from build123d import *

# Parameters (mm, degrees)
SKETCH1_R               = 10
BOSS_EXTRUDE1_DEPTH     = 25
CUT_EXTRUDE2_DEPTH      = 257.353271873
CUT_EXTRUDE2_DEPTH_BACK = 257.353271873
SKETCH3_W               = 67
SKETCH3_H               = 15


with BuildPart() as part:
    # Sketch1 → Boss-Extrude1 (new body)
    with BuildSketch(Plane.XY):
        with BuildLine():
            Line((-230, 24), (230, 24))
            ThreePointArc((230, 24), (254, 0), (230, -24))
            Line((230, -24), (-230, -24))
            ThreePointArc((-230, -24), (-254, 0), (-230, 24))
        make_face()
        with Locations((-230, 0)):
            Circle(SKETCH1_R, mode=Mode.SUBTRACT)
        with Locations(Location((230, 0, 0), (0, 0, 180))):
            Circle(SKETCH1_R, mode=Mode.SUBTRACT)
    extrude(amount=-BOSS_EXTRUDE1_DEPTH)

    # Sketch3 → Cut-Extrude2 (cut, two sides: drawn at the far end of the back side and taken through both)
    with BuildSketch(Plane(origin=(0, 0, 0), x_dir=(1, 0, 0), z_dir=(0, 1, 0)).offset(-CUT_EXTRUDE2_DEPTH_BACK)):
        with Locations((-230, 12.5)):
            Rectangle(SKETCH3_W, SKETCH3_H)
        with Locations((230, 12.5)):
            Rectangle(SKETCH3_W, SKETCH3_H)
    extrude(amount=CUT_EXTRUDE2_DEPTH + CUT_EXTRUDE2_DEPTH_BACK, mode=Mode.SUBTRACT)


solid = part.part
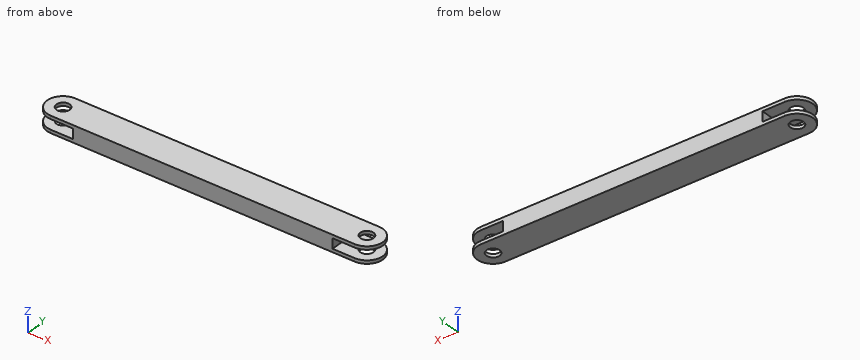
Design review of the part built by this model. Coordinates are the model's own, in mm. Round coordinates to 2 decimals unless told otherwise and drop trailing zeros. Write each loop counter-clockwise with the first axis right and the second up, starting at its lowest first coordinate (ties: lowest second). Pieces come first, ordered by that corner, then holes. Notation, with made-up numbers: (66, -26) - (70, -26) arc R32 cw to (70, 8) - close; hole circle Ø6 at (36, 51). An arc over 180 degrees is marked (long way). Return JSON: item names as keys, results as strings. Group by question number.
Item 1: For probe 1 along Z at (x, y) = (-222.5, -13); probe 2 along Y at (x, z) = (230, -22.5); probe 3 along X at (y, z) = (21.5, -5.25), list the stretches that pass through material, from the lowest coordinate up. Write a range as [from, to].
Item 2: We need section C-C on z = -9. Write out the cut boundary in (x, y).
Item 3: We need section B-B on y = 0. Write out the cut boundary in (x, z).
Item 4: We need section A-A on x = -211.5. Write out the cut boundary in (y, z).
Item 5: We need section D-D on y = 19. Write out the cut boundary in (x, z), and give its area (3 significant figures).
Item 6: Insertion check: P1, Ø10, axis at y = -8.5, z = -5, coming from the -X side; P2, Ø12, axis at x = -196.5, y = 2.5, coming from the +Z side; P3, Ø4, axis at y = 19, z = -21, coming from the -X side; P4, Ø8, axis at y = 6.5, z = -16.5, coming from the -X side. Each pin has a flat end and moves straight along its axis. Give the tip position at first contact, or say it passes through.
Model answer:
{
 "1": {"probe 1": "z = [-25, -20], [-5, 0]", "probe 2": "y = [-24, -10], [10, 24]", "probe 3": "x = [-196.5, 196.5]"},
 "2": {"outline": "(-196.5, -24) - (196.5, -24) - (196.5, 24) - (-196.5, 24) - close"},
 "3": {"outline": "(-254, -25) - (-240, -25) - (-240, -20) - (-254, -20) - close; (-254, -5) - (-240, -5) - (-240, 0) - (-254, 0) - close; (-220, -25) - (220, -25) - (220, -20) - (196.5, -20) - (196.5, -5) - (220, -5) - (220, 0) - (-220, 0) - (-220, -5) - (-196.5, -5) - (-196.5, -20) - (-220, -20) - close; (240, -25) - (254, -25) - (254, -20) - (240, -20) - close; (240, -5) - (254, -5) - (254, 0) - (240, 0) - close"},
 "4": {"outline": "(-24, -25) - (24, -25) - (24, -20) - (-24, -20) - close; (-24, -5) - (24, -5) - (24, 0) - (-24, 0) - close"},
 "5": {"outline": "(-244.66, -25) - (244.66, -25) - (244.66, -20) - (196.5, -20) - (196.5, -5) - (244.66, -5) - (244.66, 0) - (-244.66, 0) - (-244.66, -5) - (-196.5, -5) - (-196.5, -20) - (-244.66, -20) - close", "area": "10,800 mm²"},
 "6": {"P1": "stops at x = -253.74", "P2": "stops at z = 0", "P3": "stops at x = -246.94", "P4": "stops at x = -253.56"}
}
